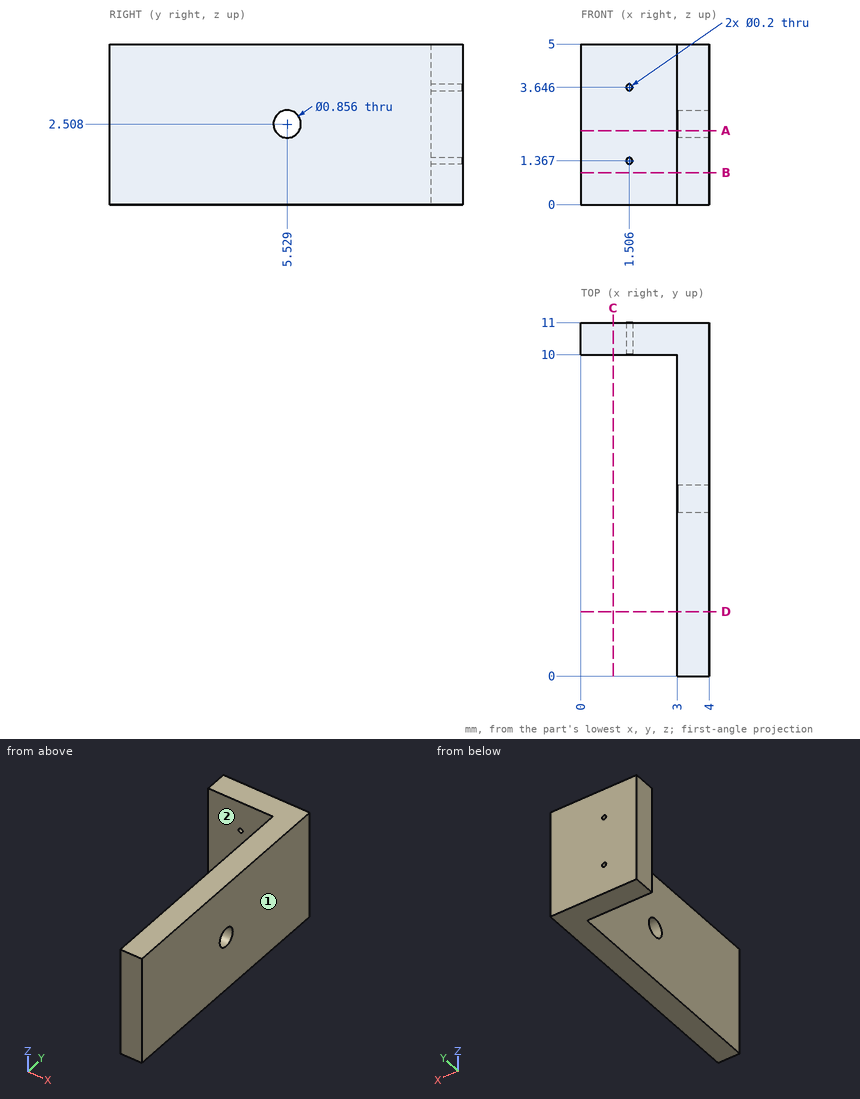
For this review, use the dimensioned drawing (mm, ordinates from the lowest corner) and the shaded views. A direction names the side the tool comes from. Round coordinates to 2 decimals unless told otherwise and drop trailing zeros. Order: outer loops, then holes, each group sorted by start corner. A loop starts at its lowest first (then second) coordinate and runs counter-clockwise, first axis right, second up. Notation, with made-up numbers: M -23,-3 L 25,-3 A17 ccw 25,22 Z; hole C 88.25,-23.5 d3. An arc over 180 degrees is marked long. Write each question's results on one line, items separated by ' | '. Start each with the question number.
1. Add section D-D (y = 2). State the section outline as (x, z) points.
2. To check wall thickness, follow L1, parallel to X at y = 5.75, z = 3.4; L2, parallel to Y at x = 0.55, z = 1.1; L3, parallel to Y at x = 3.35, z = 2.7 (1 decimal). State the ranges of each line that lie inside material, in increasing order. Write a range as [from, to].
3. Add section C-C (x = 1). State the section outline as (y, z) points.
4. Tool access review of the marked faces 1 and 2: name each direction out of +Z, -Z, +X, -X, +Y, -Y from which nothing blocks a thin tool from reaching the whole face with its end or side.
5. Add section B-B (z = 1). State the section outline as (x, y) points, then the cut area to 3 significant figures.
6. Add section A-A (z = 2.3). State the section outline as (x, y) points (1 decimal).
Output values:
1) outline: M 3,0 L 4,0 L 4,5 L 3,5 Z
2) L1: [3, 4] | L2: [10, 11] | L3: [0, 5.1], [5.9, 11]
3) outline: M 10,0 L 11,0 L 11,5 L 10,5 Z
4) face 1: +Z, -Z, +X, +Y, -Y | face 2: +Z, -Z, -X, -Y
5) outline: M 0,10 L 3,10 L 3,0 L 4,0 L 4,11 L 0,11 Z | area: 14.0 mm^2
6) outline: M 0,10 L 3,10 L 3,5.9 L 4,5.9 L 4,11 L 0,11 Z; M 3,0 L 4,0 L 4,5.2 L 3,5.2 Z
